Build history of the part. All positions in model axes, mm. Face numbers are marked on the shaded views. A direction names the side the tool comes from. Round coordinates to 2 decimals unless told otherwise and drop trailing zeros. Loops run counter-clockwise (first coordinate to the right, second up) from the corner with the lowest first, then second, coordinate; pieces in that order, holes last. Notation, with made-up numbers: (20, 15) -> (74, 15) arc R20 ccw to (74, 25) -> close; hole circle Ø9 at (18.5, 87). An arc over 180 degrees is marked (long way). Put each result on its own line as item: value. Start each with the question number.
Item 1: Flat gauge pins, fed straight in: pin 1 Ø1.5 at (y, z) = (9, -17.5) entering from +X; pin 2 Ø6 at (x, y) = (14.5, 35) entering from +Z; pin 3 Ø3 at (x, y) = (-35.5, 8.5) entering from -Z; pin 4 Ø6 at (x, y) = (45.5, 26) entering from -Z. Where does each tip first touch, or does it go through?
Item 2: Tool access for the marked faces 5, 6 and 7: list every direction of +Z, -Z, +X, -X, +Y, -Y with a clear straight run to the whole face (end or side of a thin tool).
Item 3: Pull direction Z, two halves, no side cores. Call the marked faces 1, 2, 3 and 4: +Z half, -Z half, draft (parallel to the pull), parting line (faces both ways), or undercut.
Item 4: Cut at A-A, the plane y = -8.5. List the corners of the cut face in (x, z).
Item 5: Cut at C-C, the plane y = 47.5. List the corners of the cut face in (x, z).
Item 6: Drill centre lines: probe 1 along Z at (x, y) = (0, -7); probe 2 along X at (y, z) = (-3, 0); probe 3 along Y at (x, z) = (-7, -53). Where is each one in solid material? Low to high. Write a range as [from, to].
Item 7: Cut at B-B, the plane z = 0. List the corners of the cut face in (x, y).
```python
from build123d import *

# Parameters (mm, degrees)
SKETCH1_R           = 75
SKETCH1_R_2         = 40
BOSS_EXTRUDE1_DEPTH = 3
SKETCH1_3_R         = 40
BOSS_EXTRUDE2_DEPTH = 55
SKETCH2_R           = 26
CUT_EXTRUDE1_DEPTH  = 119.127050247
FILLET1_R           = 3
CHAMFER2_SIZE       = 2
CHAMFER3_SIZE       = 2
CHAMFER4_SIZE       = 1
SKETCH3_R           = 26
BOSS_EXTRUDE3_DEPTH = 17
FILLET3_R           = 3


with BuildPart() as part:
    # Sketch1 → Boss-Extrude1 (new body)
    # profile 1 of 3: a face of its own
    with BuildSketch(Plane(origin=(0, 0, 0), x_dir=(1, 0, 0), z_dir=(0, 1, 0))):
        with Locations(Location((0, 0, 0), (0, 0, 270))):
            Circle(SKETCH1_R)
        Circle(SKETCH1_R_2, mode=Mode.SUBTRACT)
    # profile 2 of 3: a face of its own
    with BuildSketch(Plane(origin=(0, 0, 0), x_dir=(1, 0, 0), z_dir=(0, 1, 0))):
        Circle(SKETCH1_R_2)
        Polygon((0, -38.105117767), (33, -19.052558883), (33, 19.052558883), (0, 38.105117767), (-33, 19.052558883), (-33, -19.052558883), align=None, mode=Mode.SUBTRACT)
    # profile 3 of 3: a face of its own
    with BuildSketch(Plane(origin=(0, 0, 0), x_dir=(1, 0, 0), z_dir=(0, 1, 0))):
        Polygon((-33, -19.052558883), (0, -38.105117767), (33, -19.052558883), (33, 19.052558883), (0, 38.105117767), (-33, 19.052558883), align=None)
    extrude(amount=BOSS_EXTRUDE1_DEPTH)

    # Sketch1_3 → Boss-Extrude2 (add)
    with BuildSketch(Plane(origin=(0, 0, 0), x_dir=(1, 0, 0), z_dir=(0, 1, 0))):
        with Locations(Location((0, 0, 0), (0, 0, 270))):
            Circle(SKETCH1_3_R)
        Polygon((0, -38.105117767), (33, -19.052558883), (33, 19.052558883), (0, 38.105117767), (-33, 19.052558883), (-33, -19.052558883), align=None, mode=Mode.SUBTRACT)
    extrude(amount=BOSS_EXTRUDE2_DEPTH)

    # Sketch2 → Cut-Extrude1 (cut, through all)
    with BuildSketch(Plane(origin=(0, 3, 0), x_dir=(1, 0, 0), z_dir=(0, 1, 0))):
        with Locations(Location((0, 0, 0), (0, 0, 270))):
            Circle(SKETCH2_R)
    extrude(amount=-CUT_EXTRUDE1_DEPTH, mode=Mode.SUBTRACT)

    # Fillet1
    fillet1_edges = [part.edges().sort_by_distance(p)[0] for p in [
        (33, 29, 19.052558883),
        (0, 29, 38.105117767),
        (-33, 29, 19.052558883),
        (-33, 29, -19.052558883),
        (0, 29, -38.105117767),
        (33, 29, -19.052558883),
    ]]
    fillet(fillet1_edges, radius=FILLET1_R)

    # Chamfer2
    chamfer2_edges = [part.edges().sort_by_distance(p)[0] for p in [
        (16.5, 3, 28.578838325),
        (33, 3, 0),
        (16.5, 3, -28.578838325),
        (-16.5, 3, -28.578838325),
        (-33, 3, 0),
        (-16.5, 3, 28.578838325),
        (32.598076211, 3, -18.820508076),
        (0, 3, -37.641016151),
        (-32.598076211, 3, -18.820508076),
        (-32.598076211, 3, 18.820508076),
        (0, 3, 37.641016151),
        (32.598076211, 3, 18.820508076),
    ]]
    chamfer(chamfer2_edges, length=CHAMFER2_SIZE)

    # Chamfer3
    chamfer3_edges = [part.edges().sort_by_distance(p)[0] for p in [
        (0, 3, -40),
    ]]
    chamfer(chamfer3_edges, length=CHAMFER3_SIZE)

    # Chamfer4
    chamfer4_edges = [part.edges().sort_by_distance(p)[0] for p in [
        (0, 0, -75),
        (0, 3, -75),
    ]]
    chamfer(chamfer4_edges, length=CHAMFER4_SIZE)

    # Sketch3 → Boss-Extrude3 (add)
    with BuildSketch(Plane.XZ):
        Polygon((32.5, -18.763883749), (32.5, 18.763883749), (0, 37.527767497), (-32.5, 18.763883749), (-32.5, -18.763883749), (0, -37.527767497), align=None)
        with Locations(Location((0, 0, 0), (0, 0, 90))):
            Circle(SKETCH3_R, mode=Mode.SUBTRACT)
    extrude(amount=BOSS_EXTRUDE3_DEPTH)

    # Fillet3
    fillet3_edges = [part.edges().sort_by_distance(p)[0] for p in [
        (0, -8.5, -37.527767497),
        (32.5, -8.5, -18.763883749),
        (32.5, -8.5, 18.763883749),
        (0, -8.5, 37.527767497),
        (-32.5, -8.5, 18.763883749),
        (-32.5, -8.5, -18.763883749),
    ]]
    fillet(fillet3_edges, radius=FILLET3_R)


solid = part.part
```
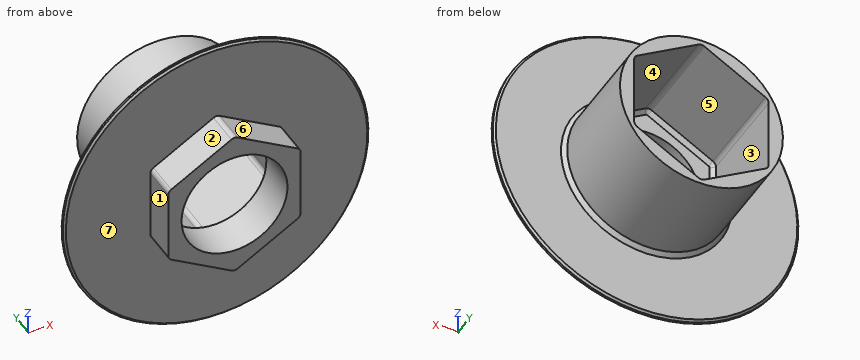
Reply:
1. pin 1: stops at x = 36.32
1. pin 2: stops at z = 38.31
1. pin 3: stops at z = -21.07
1. pin 4: passes through
2. face 5: +Y
2. face 6: +Z, +X, -Y
2. face 7: -Y
3. face 1: draft
3. face 2: +Z half
3. face 3: undercut
3. face 4: undercut
4. outline: (-32.5, -17.03) arc R3 ccw to (-31, -19.63) -> (-1.5, -36.66) arc R3 ccw to (1.5, -36.66) -> (31, -19.63) arc R3 ccw to (32.5, -17.03) -> (32.5, 17.03) arc R3 ccw to (31, 19.63) -> (1.5, 36.66) arc R3 ccw to (-1.5, 36.66) -> (-31, 19.63) arc R3 ccw to (-32.5, 17.03) -> close; hole circle Ø52 at (0, 0)
5. outline: circle Ø80 at (0, 0); hole (-33, -17.32) arc R3 ccw to (-31.5, -19.92) -> (-1.5, -37.24) arc R3 ccw to (1.5, -37.24) -> (31.5, -19.92) arc R3 ccw to (33, -17.32) -> (33, 17.32) arc R3 ccw to (31.5, 19.92) -> (1.5, 37.24) arc R3 ccw to (-1.5, 37.24) -> (-31.5, 19.92) arc R3 ccw to (-33, 17.32) -> close
6. probe 1: z = [-37.06, -26], [26, 37.06]
6. probe 2: x = [-32.5, -26], [26, 32.5]
6. probe 3: y = [0, 3]
7. outline: (-75, 1) -> (-74, 0) -> (-32.5, 0) -> (-32.5, -17) -> (-26, -17) -> (-26, 3) -> (-31, 3) -> (-33, 5) -> (-33, 55) -> (-40, 55) -> (-40, 5) -> (-42, 3) -> (-74, 3) -> (-75, 2) -> close; (26, -17) -> (32.5, -17) -> (32.5, 0) -> (74, 0) -> (75, 1) -> (75, 2) -> (74, 3) -> (42, 3) -> (40, 5) -> (40, 55) -> (33, 55) -> (33, 5) -> (31, 3) -> (26, 3) -> close
